Input: part model. Units: mm. Frame: model coordinates. Face numbers are marked on the shaded views. A direction names the side the tool comes from. Round coordinates to 2 decimals unless told otherwise and drop trailing zeros. Order: outer loops, then holes, each group sorted by start corner. A loop starts at its lowest first (then second) coordinate and runs counter-clockwise, first axis right, second up. Notation, with made-up numbers: (56, -32.5) -> (95, -32.5) arc R12 ccw to (95, -9.5) -> close; hole circle Ø4 at (84, 42.25). An arc over 180 degrees is marked (long way). Answer as CSV lines item,"result". Start each with the question number.
1) Section query D-D, the plane z = -22. Output: boundary loops of the cut face in (x, y).
2) First-contact query: P1, Ø6, axis at x = 14.5, y = 6.5, coming from the -Z side; P2, Ø6, axis at x = 2.5, z = -3, coming from the -Y side; P3, Ø5, axis at x = -20.5, y = 6, coming from the -Z side. Flat tips, straight axial feed; report the tip coordinate or a pass-through.
3) Mould query, pull axis Z, two halves, no side actions, for the marked faces 1, 2 and 3. Classes: +Z half, -Z half, draft (parallel to the pull), parting line (faces both ways), or undercut.
4) Section query C-C, the plane y = 7.75. Output: boundary loops of the cut face in (x, z).
5) Line query: L1, parallel to Z at x = 6.5, y = 6.75; L2, parallel to Y at x = -24, z = 1.5; L3, parallel to X at y = 5, z = -9. Output: solid intervals per line, ascending.
6) Access query for the marked faces 4, 5, 6 and 7. Directions: +Z, -Z, +X, -X, +Y, -Y. A direction counts if a zero-diameter tool reaches every point of the face in a straight line with its end or side. Return the directions, or none.
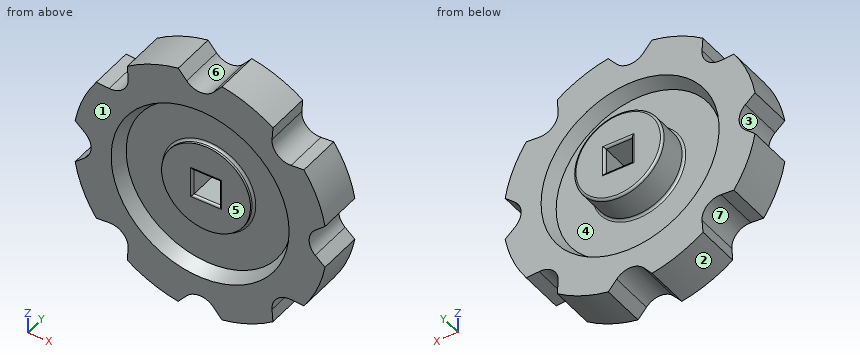
```python
from build123d import *

# Parameters (mm, degrees)
SKETCH_1_W          = 10
SKETCH_1_H          = 7
SKETCH_1_H_2        = 1
FILLET_3_R          = 0.5
FILLET_4_R          = 0.5
CUT_EXTRUDE_1_DEPTH = 10
CUT_EXTRUDE_2_REACH = 14
SKETCH_5_W          = 6
SKETCH_5_H          = 6
FILLET_5_R          = 0.5
FILLET_6_R          = 0.5


with BuildPart() as part:
    # Эскиз1 → Повернуть1 (revolve)
    with BuildSketch(Plane.XY):
        Polygon((20, 4), (20, 2), (20, 0), (20, -3), (28.5, -3), (28.5, 7), (20, 7), align=None)
        Polygon((20, 0), (20, 2), (20, 4), (18.625227292, 4), (10, 4), (0, 4), (0, 0), (10, 0), (18.625227292, 0), align=None)
        with Locations((5, 7.5)):
            Rectangle(SKETCH_1_W, SKETCH_1_H)
        with Locations((5, -0.5)):
            Rectangle(SKETCH_1_W, SKETCH_1_H_2)
        Polygon((18.625227292, 4), (20, 4), (20, 7), align=None)
        Polygon((20, -3), (20, 0), (18.625227292, 0), align=None)
    revolve(axis=Axis((0, 0, 0), (0, 1, 0)))

    # Скругление3
    fillet_3_edges = [part.edges().sort_by_distance(p)[0] for p in [
        (-10, 4, 0),
    ]]
    fillet(fillet_3_edges, radius=FILLET_3_R)

    # Скругление4
    fillet_4_edges = [part.edges().sort_by_distance(p)[0] for p in [
        (-10, 0, 0),
    ]]
    fillet(fillet_4_edges, radius=FILLET_4_R)

    # Эскиз4 → Вырез-Вытянуть1 (cut)
    with BuildSketch(Plane(origin=(0, 7, 0), x_dir=(1, 0, 0), z_dir=(0, 1, 0))):
        with BuildLine():
            Line((-3.032652989, 25.883771919), (-8.753058696, 32.499672333))
            Line((-8.753058696, 32.499672333), (8.739316139, 32.499672333))
            Line((8.739316139, 32.499672333), (3.018910432, 25.883771919))
            ThreePointArc((3.018910432, 25.883771919), (-0.006871279, 24.499999172), (-3.032652989, 25.883771919))
        make_face()
        with BuildLine():
            Line((16.791391533, 29.170085853), (29.160368398, 16.801108988))
            Line((29.160368398, 16.801108988), (20.437282685, 16.167898608))
            ThreePointArc((20.437282685, 16.167898608), (17.319256826, 17.328974281), (16.158181153, 20.44700014))
            Line((16.158181153, 20.44700014), (16.791391533, 29.170085853))
        make_face()
        with BuildLine():
            Line((32.499672333, 8.753058696), (32.499672333, -8.739316139))
            Line((32.499672333, -8.739316139), (25.883771919, -3.018910432))
            ThreePointArc((25.883771919, -3.018910432), (24.499999172, 0.006871279), (25.883771919, 3.032652989))
            Line((25.883771919, 3.032652989), (32.499672333, 8.753058696))
        make_face()
        with BuildLine():
            Line((29.170085853, -16.791391533), (16.801108988, -29.160368398))
            Line((16.801108988, -29.160368398), (16.167898608, -20.437282685))
            ThreePointArc((16.167898608, -20.437282685), (17.328974281, -17.319256826), (20.44700014, -16.158181153))
            Line((20.44700014, -16.158181153), (29.170085853, -16.791391533))
        make_face()
        with BuildLine():
            Line((8.753058696, -32.499672333), (-8.739316139, -32.499672333))
            Line((-8.739316139, -32.499672333), (-3.018910432, -25.883771919))
            ThreePointArc((-3.018910432, -25.883771919), (0.006871279, -24.499999172), (3.032652989, -25.883771919))
            Line((3.032652989, -25.883771919), (8.753058696, -32.499672333))
        make_face()
        with BuildLine():
            Line((-16.791391533, -29.170085853), (-29.160368398, -16.801108988))
            Line((-29.160368398, -16.801108988), (-20.437282685, -16.167898608))
            ThreePointArc((-20.437282685, -16.167898608), (-17.319256826, -17.328974281), (-16.158181153, -20.44700014))
            Line((-16.158181153, -20.44700014), (-16.791391533, -29.170085853))
        make_face()
        with BuildLine():
            Line((-32.499672333, -8.753058696), (-32.499672333, 8.739316139))
            Line((-32.499672333, 8.739316139), (-25.883771919, 3.018910432))
            ThreePointArc((-25.883771919, 3.018910432), (-24.499999172, -0.006871279), (-25.883771919, -3.032652989))
            Line((-25.883771919, -3.032652989), (-32.499672333, -8.753058696))
        make_face()
        with BuildLine():
            Line((-29.170085853, 16.791391533), (-16.801108988, 29.160368398))
            Line((-16.801108988, 29.160368398), (-16.167898608, 20.437282685))
            ThreePointArc((-16.167898608, 20.437282685), (-17.328974281, 17.319256826), (-20.44700014, 16.158181153))
            Line((-20.44700014, 16.158181153), (-29.170085853, 16.791391533))
        make_face()
    extrude(amount=-CUT_EXTRUDE_1_DEPTH, mode=Mode.SUBTRACT)

    # Эскиз5 → Вырез-Вытянуть2 (cut, up to next)
    with BuildSketch(Plane.XZ.offset(1), mode=Mode.PRIVATE) as cut_extrude_2_sk1:
        Rectangle(SKETCH_5_W, SKETCH_5_H)
    cut_extrude_2_tool1 = extrude(cut_extrude_2_sk1.sketch, amount=-CUT_EXTRUDE_2_REACH, mode=Mode.PRIVATE) & part.part
    add(cut_extrude_2_tool1.solids().sort_by_distance((0, -1, 0))[0], mode=Mode.SUBTRACT)

    # Скругление5
    fillet_5_edges = [part.edges().sort_by_distance(p)[0] for p in [
        (3, -1, 0),
        (0, -1, 3),
        (-3, -1, 0),
        (0, -1, -3),
        (0, 11, 3),
        (3, 11, 0),
        (0, 11, -3),
        (-3, 11, 0),
    ]]
    fillet(fillet_5_edges, radius=FILLET_5_R)

    # Скругление6
    fillet_6_edges = [part.edges().sort_by_distance(p)[0] for p in [
        (-10, 11, 0),
    ]]
    fillet(fillet_6_edges, radius=FILLET_6_R)


solid = part.part
```
Findings:
1,outline,"(-16.28, -3) -> (16.27, -3) -> (16.27, 7) -> (-16.28, 7) -> close"
2,P1,"stops at z = -26.08"
2,P2,"stops at y = -1"
2,P3,"stops at z = -16.78"
3,face 1,"draft"
3,face 2,"-Z half"
3,face 3,"undercut"
4,outline,"circle Ø20 at (0, 0); hole (-3, -3) -> (3, -3) -> (3, 3) -> (-3, 3) -> close"
5,L1,"z = -27.75 to -18.79, -7.6 to 7.6, 18.79 to 27.75"
5,L2,"y = -3 to 7"
5,L3,"x = -27.04 to -16.83, -4.36 to 4.36, 16.83 to 27.04"
6,face 4,"+Y"
6,face 5,"-Y"
6,face 6,"+Z, +Y, -Y"
6,face 7,"+Y, -Y"
